Can you work these out from the drawing? Everything is in mm from the part's minimum corner. Round coordinates to 2 decimals unless told otherwise and drop trailing zeros. Loops run counter-clockwise (first coordinate to the right, second up) from the corner with the lowest first, then second, coordinate; pieces in that order, holes last. Notation, with made-up numbers: (18.5, 83.25) -> (66.5, 83.25) arc R13 cw to (66.5, 93.25) -> close; hole circle Ø6 at (51.5, 22). An arc over 180 degrees is marked (long way). One line per item, written item: value.
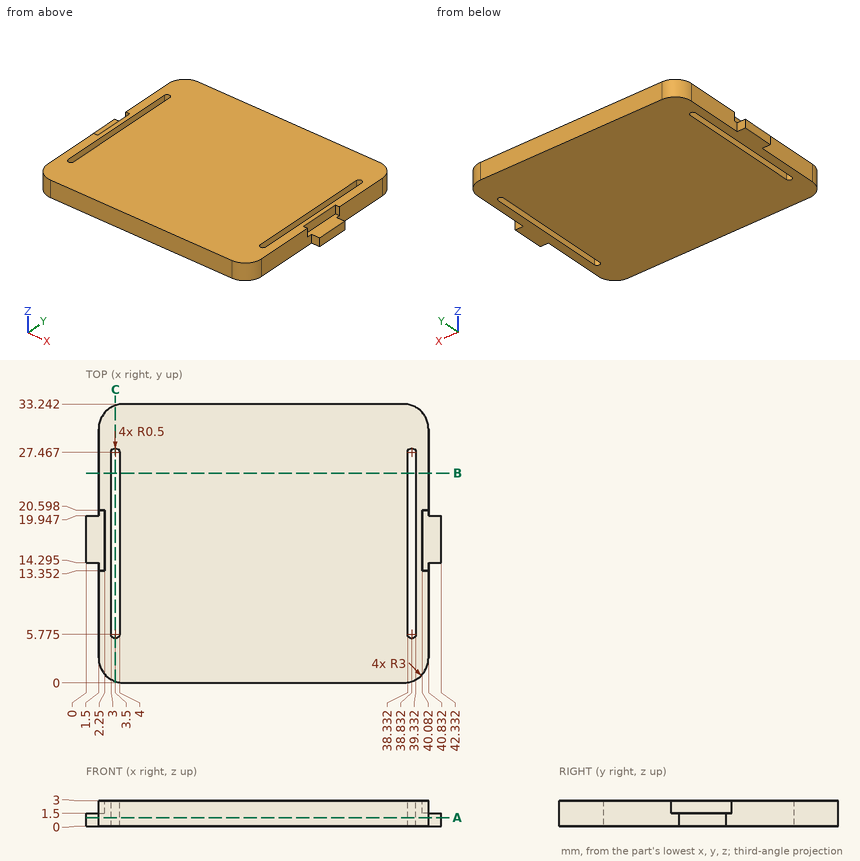
Item 1: Will these pins go through, and if not, where does the flat tip stop? pin 1 Ø1.6 at (x, z) = (42, 0.5) entering from -Y (1 decimal); pin 2 Ø0.6 at (x, z) = (40.5, 2) entering from -Y; pin 3 Ø1.5 at (y, z) = (13, 2) entering from +X.
Output:
pin 1: stops at y = 14.3
pin 2: stops at y = 1.16
pin 3: stops at x = 40.83
Item 2: If we section it at B-B on y = 25: List the corners of the cut face in (x, z) for me, plus the area to 3 significant figures.
Output:
outline: (1.5, 0) -> (3, 0) -> (3, 3) -> (1.5, 3) -> close; (4, 0) -> (38.33, 0) -> (38.33, 3) -> (4, 3) -> close; (39.33, 0) -> (40.83, 0) -> (40.83, 3) -> (39.33, 3) -> close
area: 112 mm²
Item 3: If we section it at A-A on z = 1: List the corners of the cut face in (x, y) for me (1 decimal), plus the area to 3 significant figures.
Output:
outline: (0, 14.3) -> (1.5, 14.3) -> (1.5, 3) arc R3 ccw to (4.5, 0) -> (37.8, 0) arc R3 ccw to (40.8, 3) -> (40.8, 14.3) -> (42.3, 14.3) -> (42.3, 19.9) -> (40.8, 19.9) -> (40.8, 30.2) arc R3 ccw to (37.8, 33.2) -> (4.5, 33.2) arc R3 ccw to (1.5, 30.2) -> (1.5, 19.9) -> (0, 19.9) -> close; hole (3, 5.8) arc R0.5 ccw to (4, 5.8) -> (4, 27.5) arc R0.5 ccw to (3, 27.5) -> close; hole (38.3, 5.8) arc R0.5 ccw to (39.3, 5.8) -> (39.3, 27.5) arc R0.5 ccw to (38.3, 27.5) -> close
area: 1,270 mm²
Item 4: If we section it at C-C on x = 3.5: List the corners of the cut face in (y, z) for me (1 decimal), plus the area to 3 significant figures.
Output:
outline: (0.2, 0) -> (5.3, 0) -> (5.3, 3) -> (0.2, 3) -> close; (28, 0) -> (33.1, 0) -> (33.1, 3) -> (28, 3) -> close
area: 30.6 mm²
Item 5: I need wall thicknesses on line 1 (X direction, y = 11, z = 2.6); line 2 (X direction, y = 18.5, z = 0.55); line 3 (X direction, y = 29, z = 1.4). Which ranges of each line are inside material? Lowest first, please. Write a range as from..to.
Output:
line 1: x = 1.5..3, 4..38.33, 39.33..40.83
line 2: x = 0..3, 4..38.33, 39.33..42.33
line 3: x = 1.5..40.83
